Model file for the job. Use its own axes, mm. A direction names the side the tool comes from. Give positions to 0.01 mm unless a question says otherwise; leave off trailing zeros. Order: outer loops, then holes, each group sorted by start corner. A loop starts at its lowest first (then second) coordinate and runs counter-clockwise, first axis right, second up. Notation, with made-up numbers: M 88.25,55.5 L 147.25,55.5 A36 cw 147.25,93.5 Z; hole C 38,26 d1. An arc over 180 degrees is marked long. Return JSON: item names as keys, results as strings. Group by question number.
1. Pin check, flat tips, straight feed: pin 1 (3 mm diameter, centred on x = -2, y = 5.5, fed in from +Z); pin 2 (1 mm diameter, centred on x = 2.5, z = -8.5, fed in from +Y); pin 3 (2 mm diameter, centred on x = 0.45, z = 0, fed in from -Y); pin 4 (1.5 mm diameter, centred on x = 9, z = -5.5, fed in from +Y). Stop position of each tip, or through.
2. Slice it at C-C on z = -8.55. List the corners of the cut face in (x, y), then the cut area to 3 significant figures.
3. 3-axis set-ups, long thin cutter, end or side, ignore diameter. For faces 1 (the face through (-6.324, 9.99, 1.096)), 2 (the face through (1.9, 2.5, -8.6)), 3 (the face through (-9, 1.7, -1.6)): which of +Z, -Z, +X, -X, +Y, -Y reach the whole face in a straight line?
4. Two-plate mould, pull along Z, no slides. Class faces 4 (the face through (2, 2, -8.1)), 5 (the face through (15.765, 0.493, 1.598)), 6 (the face through (-15.765, 0.493, -1.598)): released by +Z, released by -Z, zero draft, split by the parting line, or undercut.
5. Slice it at B-B on y = 1.5. List the corners of the cut face in (x, z).
6. Slice it at D-D on z = 8.55. List the corners of the cut face in (x, y).
7. Wall check: probe 1 along X at (y, z) = (0.3, 0); probe 2 along Z at (x, y) = (-6, 1.5); probe 3 along X at (y, z) = (4.5, -0.5). Give the ranges that are in metal, low to high. Write a range as [from, to].
from build123d import *
from OCP.BRepFilletAPI import BRepFilletAPI_MakeChamfer

# Parameters (mm, degrees)
ESQUISSE1_R        = 1.25
BOSS_EXTRU_1_DEPTH = 1
BOSS_EXTRU_2_DEPTH = 9.2
CONG_1_R           = 0.7
BOSS_EXTRU_3_DEPTH = 1.4
CHANFREIN1_SIZE    = 1.4
CHANFREIN1_SIZE_2  = 1.2
BOSS_EXTRU_4_DEPTH = 1.5


with BuildPart() as part:
    # Esquisse1 → Boss.-Extru.1 (new body)
    with BuildSketch(Plane(origin=(0, 0, 0), x_dir=(1, 0, 0), z_dir=(0, 1, 0))):
        with BuildLine():
            Line((-11, -9), (7.435028843, -9))
            ThreePointArc((7.435028843, -9), (8.58307914, -8.771638598), (9.556349186, -8.121320344))
            Line((9.556349186, -8.121320344), (15.121320344, -2.556349186))
            ThreePointArc((15.121320344, -2.556349186), (15.771638598, -1.58307914), (16, -0.435028843))
            Line((16, -0.435028843), (16, 4))
            ThreePointArc((16, 4), (14.535533906, 7.535533906), (11, 9))
            Line((11, 9), (-7.435028843, 9))
            ThreePointArc((-7.435028843, 9), (-8.58307914, 8.771638598), (-9.556349186, 8.121320344))
            Line((-9.556349186, 8.121320344), (-15.121320344, 2.556349186))
            ThreePointArc((-15.121320344, 2.556349186), (-15.771638598, 1.58307914), (-16, 0.435028843))
            Line((-16, 0.435028843), (-16, -4))
            ThreePointArc((-16, -4), (-14.535533906, -7.535533906), (-11, -9))
        make_face()
        with Locations(Location((0.45, 0, 0), (0, 0, 270))):
            Circle(ESQUISSE1_R, mode=Mode.SUBTRACT)
    extrude(amount=BOSS_EXTRU_1_DEPTH)

    # Esquisse2 → Boss.-Extru.2 (add)
    with BuildSketch(Plane(origin=(0, 1, 0), x_dir=(1, 0, 0), z_dir=(0, 1, 0))):
        with BuildLine():
            Line((-11.062539674, -1.308147545), (-6.042081528, 3.712310601))
            ThreePointArc((-6.042081528, 3.712310601), (-3.637918472, 3.712310601), (-3.637918472, 1.308147545))
            Line((-3.637918472, 1.308147545), (-8.658376618, -3.712310601))
            ThreePointArc((-8.658376618, -3.712310601), (-11.062539674, -3.712310601), (-11.062539674, -1.308147545))
        make_face()
        with BuildLine():
            Line((4.517002179, -1.308147545), (9.537460326, 3.712310601))
            ThreePointArc((9.537460326, 3.712310601), (11.941623382, 3.712310601), (11.941623382, 1.308147545))
            Line((11.941623382, 1.308147545), (6.921165235, -3.712310601))
            ThreePointArc((6.921165235, -3.712310601), (4.517002179, -3.712310601), (4.517002179, -1.308147545))
        make_face()
    extrude(amount=BOSS_EXTRU_2_DEPTH)

    # Congé1
    cong_1_edges = [part.edges().sort_by_distance(p)[0] for p in [
        (-11.062539674, 10.2, 3.712310601),
        (-6.148147545, 10.2, 1.202081528),
        (-3.637918472, 10.2, -3.712310601),
        (-8.552310601, 10.2, -1.202081528),
        (4.517002179, 10.2, 3.712310601),
        (9.431394308, 10.2, 1.202081528),
        (11.941623382, 10.2, -3.712310601),
        (7.027231252, 10.2, -1.202081528),
    ]]
    fillet(cong_1_edges, radius=CONG_1_R)

    # Esquisse3 → Boss.-Extru.3 (add)
    with BuildSketch(Plane(origin=(0, 1, 0), x_dir=(1, 0, 0), z_dir=(0, 1, 0))):
        with BuildLine():
            Line((-11.911067812, -0.459619408), (-6.890609665, 4.560838739))
            ThreePointArc((-6.890609665, 4.560838739), (-2.789390335, 4.560838739), (-2.789390335, 0.459619408))
            Line((-2.789390335, 0.459619408), (-7.809848481, -4.560838739))
            ThreePointArc((-7.809848481, -4.560838739), (-11.911067812, -4.560838739), (-11.911067812, -0.459619408))
        make_face()
        with BuildLine():
            Line((3.668474042, -0.459619408), (8.688932188, 4.560838739))
            ThreePointArc((8.688932188, 4.560838739), (12.790151519, 4.560838739), (12.790151519, 0.459619408))
            Line((12.790151519, 0.459619408), (7.769693373, -4.560838739))
            ThreePointArc((7.769693373, -4.560838739), (3.668474042, -4.560838739), (3.668474042, -0.459619408))
        make_face()
    extrude(amount=BOSS_EXTRU_3_DEPTH)

    # Chanfrein1
    chanfrein1_edges_1 = [part.edges().sort_by_distance(p)[0] for p in [
        (12.790151519, 2.4, -4.560838739),
    ]]
    chanfrein1_side_1 = [part.faces().sort_by_distance(p)[0] for p in [
        (12.790151519, 2.376, -4.560838739),
    ]]
    chanfrein1_edges_2 = [part.edges().sort_by_distance(p)[0] for p in [
        (6.178703115, 2.4, -2.050609665),
    ]]
    chanfrein1_side_2 = [part.faces().sort_by_distance(p)[0] for p in [
        (6.178703115, 2.376, -2.050609665),
    ]]
    chanfrein1_edges_3 = [part.edges().sort_by_distance(p)[0] for p in [
        (3.668474042, 2.4, 4.560838739),
    ]]
    chanfrein1_side_3 = [part.faces().sort_by_distance(p)[0] for p in [
        (3.668474042, 2.376, 4.560838739),
    ]]
    chanfrein1_edges_4 = [part.edges().sort_by_distance(p)[0] for p in [
        (10.279922446, 2.4, 2.050609665),
    ]]
    chanfrein1_side_4 = [part.faces().sort_by_distance(p)[0] for p in [
        (10.279922446, 2.376, 2.050609665),
    ]]
    chanfrein1_edges_5 = [part.edges().sort_by_distance(p)[0] for p in [
        (-2.789390335, 2.4, -4.560838739),
    ]]
    chanfrein1_side_5 = [part.faces().sort_by_distance(p)[0] for p in [
        (-2.789390335, 2.376, -4.560838739),
    ]]
    chanfrein1_edges_6 = [part.edges().sort_by_distance(p)[0] for p in [
        (-9.400838739, 2.4, -2.050609665),
    ]]
    chanfrein1_side_6 = [part.faces().sort_by_distance(p)[0] for p in [
        (-9.400838739, 2.376, -2.050609665),
    ]]
    chanfrein1_edges_7 = [part.edges().sort_by_distance(p)[0] for p in [
        (-11.911067812, 2.4, 4.560838739),
    ]]
    chanfrein1_side_7 = [part.faces().sort_by_distance(p)[0] for p in [
        (-11.911067812, 2.376, 4.560838739),
    ]]
    chanfrein1_edges_8 = [part.edges().sort_by_distance(p)[0] for p in [
        (-5.299619408, 2.4, 2.050609665),
    ]]
    chanfrein1_side_8 = [part.faces().sort_by_distance(p)[0] for p in [
        (-5.299619408, 2.376, 2.050609665),
    ]]
    chanfrein1 = BRepFilletAPI_MakeChamfer(part.part.solid().wrapped)
    for e in chanfrein1_edges_1:
        chanfrein1.Add(CHANFREIN1_SIZE - 0.0001, CHANFREIN1_SIZE_2 - 0.0001, e.wrapped, chanfrein1_side_1[0].wrapped)
    for e in chanfrein1_edges_2:
        chanfrein1.Add(CHANFREIN1_SIZE - 0.0001, CHANFREIN1_SIZE_2 - 0.0001, e.wrapped, chanfrein1_side_2[0].wrapped)
    for e in chanfrein1_edges_3:
        chanfrein1.Add(CHANFREIN1_SIZE - 0.0001, CHANFREIN1_SIZE_2 - 0.0001, e.wrapped, chanfrein1_side_3[0].wrapped)
    for e in chanfrein1_edges_4:
        chanfrein1.Add(CHANFREIN1_SIZE - 0.0001, CHANFREIN1_SIZE_2 - 0.0001, e.wrapped, chanfrein1_side_4[0].wrapped)
    for e in chanfrein1_edges_5:
        chanfrein1.Add(CHANFREIN1_SIZE - 0.0001, CHANFREIN1_SIZE_2 - 0.0001, e.wrapped, chanfrein1_side_5[0].wrapped)
    for e in chanfrein1_edges_6:
        chanfrein1.Add(CHANFREIN1_SIZE - 0.0001, CHANFREIN1_SIZE_2 - 0.0001, e.wrapped, chanfrein1_side_6[0].wrapped)
    for e in chanfrein1_edges_7:
        chanfrein1.Add(CHANFREIN1_SIZE - 0.0001, CHANFREIN1_SIZE_2 - 0.0001, e.wrapped, chanfrein1_side_7[0].wrapped)
    for e in chanfrein1_edges_8:
        chanfrein1.Add(CHANFREIN1_SIZE - 0.0001, CHANFREIN1_SIZE_2 - 0.0001, e.wrapped, chanfrein1_side_8[0].wrapped)
    add(Compound.cast(chanfrein1.Shape()), mode=Mode.REPLACE)  # a hair under: the kernel refuses the full size

    # Esquisse4 → Boss.-Extru.4 (add)
    with BuildSketch(Plane(origin=(0, 1, 0), x_dir=(1, 0, 0), z_dir=(0, 1, 0))):
        with BuildLine():
            Line((-6.667514421, 9), (10.232485579, 9))
            ThreePointArc((10.232485579, 9), (10.682485579, 8.55), (10.232485579, 8.1))
            Line((10.232485579, 8.1), (-6.667514421, 8.1))
            ThreePointArc((-6.667514421, 8.1), (-7.117514421, 8.55), (-6.667514421, 9))
        make_face()
        with BuildLine():
            Line((-11.132485579, -8.1), (7.567514421, -8.1))
            ThreePointArc((7.567514421, -8.1), (8.017514421, -8.55), (7.567514421, -9))
            Line((7.567514421, -9), (-11.132485579, -9))
            ThreePointArc((-11.132485579, -9), (-11.582485579, -8.55), (-11.132485579, -8.1))
        make_face()
    extrude(amount=BOSS_EXTRU_4_DEPTH)


solid = part.part
Result:
{
 "1": {"pin 1": "stops at z = -1.46", "pin 2": "stops at y = 2.5", "pin 3": "passes through", "pin 4": "stops at y = 1.22"},
 "2": {"outline": "M -9.02,0 L 13.07,0 L 13.07,1 L 10.68,1 L 10.68,2.5 L -7.12,2.5 L -7.12,1 L -9.02,1 Z", "area": "48.8 mm2"},
 "3": {"face 1": "+Z, +Y", "face 2": "-Z, +X, -X, +Y", "face 3": "-X, +Y"},
 "4": {"face 4": "undercut", "face 5": "released by +Z", "face 6": "released by -Z"},
 "5": {"outline": "M -11.61,0.76 L -6.59,-4.26 A2.47 ccw -3.09,-0.76 L -8.11,4.26 A2.47 ccw Z; M -11.13,8.1 L 7.57,8.1 A0.45 ccw 7.57,9 L -11.13,9 A0.45 ccw Z; M -6.67,-9 L 10.23,-9 A0.45 ccw 10.23,-8.1 L -6.67,-8.1 A0.45 ccw Z; M 3.97,0.76 L 8.99,-4.26 A2.47 ccw 12.49,-0.76 L 7.47,4.26 A2.47 ccw Z"},
 "6": {"outline": "M -13.07,0 L 9.02,0 L 9.02,1 L 8.02,1 L 8.02,2.5 L -11.58,2.5 L -11.58,1 L -13.07,1 Z"},
 "7": {"probe 1": "x = [-16, -0.8], [1.7, 16]", "probe 2": "z = [-9, -8.1], [-4.69, 2.15], [8.1, 9]", "probe 3": "x = [-9.25, -4.45], [6.33, 11.13]"}
}
